Geometry check sheet. Reference: the model listing, model coordinates, mm. A direction names the side the tool comes from. Coordinates: 2 decimals unless noted, no trailing zeros. Order: outer loops, then holes, each group sorted by start corner. A loop starts at its lowest first (then second) coordinate and runs counter-clockwise, first axis right, second up. Notation, with made-up numbers: (29, 64) -> (43, 64) arc R21 ccw to (43, 88) -> close; hole circle Ø2 at (-22, 75). An arc over 180 degrees is marked (long way). Answer in a Markdown table with one row per item. Add a question column.
```python
from build123d import *

# Parameters (mm, degrees)
PAD_DEPTH = 5


with BuildPart() as part:
    # Sketch059 → Pad (new body)
    with BuildSketch(Plane.XY):
        with BuildLine():
            Line((-4.25, 11.6), (-4.82735, 12.6))
            Line((-4.82735, 12.6), (-13.17265, 12.6))
            Line((-13.17265, 12.6), (-13.75, 11.6))
            Line((-13.75, 11.6), (-13.75, 7.6))
            Line((-13.75, 7.6), (-160.5, 7.6))
            Line((-160.5, 7.6), (-160.5, 11.6))
            Line((-160.5, 11.6), (-161.07735, 12.6))
            Line((-161.07735, 12.6), (-168.92265, 12.6))
            Line((-168.92265, 12.6), (-169.5, 11.6))
            Line((-169.5, 11.6), (-169.5, 7.6))
            Line((-169.5, 7.6), (-231.02, 7.6))
            Line((-231.02, 7.6), (-231.02, 2.6))
            Line((-231.02, 2.6), (-229, 2.6))
            Line((-229, 2.6), (-229, 2.1))
            Line((-229, 2.1), (-229.75, 2.1))
            Line((-229.75, 2.1), (-229.75, -0.4))
            Line((-229.75, -0.4), (-231.02, -0.4))
            Line((-231.02, -0.4), (-231.02, -2.4))
            Line((-231.02, -2.4), (-233.98, -2.4))
            Line((-233.98, -2.4), (-233.98, -0.4))
            Line((-233.98, -0.4), (-235.25, -0.4))
            Line((-235.25, -0.4), (-235.25, 2.1))
            Line((-235.25, 2.1), (-236, 2.1))
            Line((-236, 2.1), (-236, 2.6))
            Line((-236, 2.6), (-233.98, 2.6))
            Line((-233.98, 2.6), (-233.98, 7.6))
            Line((-233.98, 7.6), (-241, 7.6))
            Line((-241, 7.6), (-241, 3.6))
            Line((-241, 3.6), (-250.8, 3.6))
            Line((-250.8, 3.6), (-250.8, 3.1))
            Line((-250.8, 3.1), (-255.2, 3.1))
            Line((-255.2, 3.1), (-255.2, 5.6))
            Line((-255.2, 5.6), (-259.093151, 5.6))
            Line((-259.093151, 5.6), (-259.093151, 7.6))
            Line((-259.093151, 7.6), (-290, 7.6))
            Line((-290, 7.6), (-290, 11.6))
            Line((-290, 11.6), (-290.57735, 12.6))
            Line((-290.57735, 12.6), (-298.92265, 12.6))
            Line((-298.92265, 12.6), (-299.5, 11.6))
            Line((-299.5, 11.6), (-299.5, 7.6))
            Line((-299.5, 7.6), (-298.5, 7.6))
            Line((-298.5, 7.6), (-292.5, 1.6))
            Line((-292.5, 1.6), (-292.5, -8.4))
            Line((-292.5, -8.4), (-297.5, -8.4))
            Line((-297.5, -8.4), (-297.5, -15.4))
            Line((-289.270832, -15.4), (-297.5, -15.4))
            Line((-289.270832, -13.4), (-289.270832, -15.4))
            ThreePointArc((-287.270832, -11.4), (-288.685046, -11.985786), (-289.270832, -13.4))
            Line((-287.270832, -11.4), (-243.200536, -11.4))
            ThreePointArc((-239.738833, -12.018283), (-241.442294, -11.555784), (-243.200536, -11.4))
            ThreePointArc((-239.738833, -12.018283), (-232.5, -13.311187), (-225.261167, -12.018283))
            ThreePointArc((-221.799464, -11.4), (-223.557706, -11.555784), (-225.261167, -12.018283))
            Line((-221.799464, -11.4), (-6, -11.4))
            Line((-6, -11.4), (0, -5.4))
            Line((0, -5.4), (0, 0))
            Line((0, 0), (20, 0))
            Line((20, 0), (20, 7.6))
            Line((20, 7.6), (-4.25, 7.6))
            Line((-4.25, 7.6), (-4.25, 11.6))
        make_face()
    extrude(amount=PAD_DEPTH)


solid = part.part
```
(1) Cross-section at A-A (x = -9). Enter the section's corners in (y, z).
(2) Cross-section at B-B (x = -136.5). Enter the section's corners in (y, z), plus the area to 3 significant figures.
(3) Go/stop test with flat-tipped pins: P1, Ø3, axis at x = -252.5, z = 4, coming from the -Y side; P2, Ø1.2, axis at y = 10, z = 3, coming from the +X side; P3, Ø1.5, axis at x = -199, z = 2, coming from the +Y side. Record where each tip stops, or that it passes through.
(4) Scan lines: line 1 along X through (y, z) = (8.75, 4.35); line 2 along X through (y, z) = (4, 2.7); line 3 along X through (y, z) = (-0.25, 0.5). Record each from-to range of solid material in increasing order.
(5) Mould release check, pull along Y, two halves, no side actions. Record for faces 4 (the face through (-295.5, 4.6, 2.5)), 5 (the face through (8, 7.6, 2)), 6 (the face through (-293, -15.4, 2)): +Y half, -Y half, draft (parallel to the pull), parting line (faces both ways), or undercut.
(6) Access from +Z, -Z, +X, -X, +Y, -Y to the whole of each face (thin tool, end or side, straight path). Record for faces 1 (the face through (-292.5, -3, 2)), 2 (the face through (-297.5, -12, 2)), 3 (the face through (-200, 7.6, 2)).
Checks:
| question | item | result |
|---|---|---|
| 1 | outline | (-11.4, 0) -> (12.6, 0) -> (12.6, 5) -> (-11.4, 5) -> close |
| 2 | outline | (-11.4, 0) -> (7.6, 0) -> (7.6, 5) -> (-11.4, 5) -> close |
| 2 | area | 95.0 mm² |
| 3 | P1 | y = -11.4 |
| 3 | P2 | x = -4.25 |
| 3 | P3 | y = 7.6 |
| 4 | line 1 | -299.5 to -290, -169.5 to -160.5, -13.75 to -4.25 |
| 4 | line 2 | -294.9 to -255.2, -241 to -233.98, -231.02 to 20 |
| 4 | line 3 | -292.5 to -235.25, -229.75 to 0 |
| 5 | face 4 | undercut |
| 5 | face 5 | +Y half |
| 5 | face 6 | -Y half |
| 6 | face 1 | +Z, -Z, -X |
| 6 | face 2 | +Z, -Z, -X, -Y |
| 6 | face 3 | +Z, -Z, +Y |
